Read the model definition and answer for the solid it produces. Units are mm, in the model's axes. A direction names the side the tool comes from. Round coordinates to 2 decimals unless told otherwise and drop trailing zeros. Write each loop counter-clockwise with the first axis right and the second up, starting at its lowest first coordinate (ties: lowest second). Pieces come first, ordered by that corner, then holes. Notation, with made-up numbers: (89.5, -12.75) -> (136.5, -12.75) arc R24 cw to (136.5, 25.25) -> close; hole circle Ø1 at (-20.75, 84.25). An arc over 180 degrees is marked (long way). Return JSON: item names as keys, results as strings.
from build123d import *

# Parameters (mm, degrees)
BOSS_EXTRUDE1_DEPTH = 15
SKETCH2_R           = 1.65
SKETCH2_W           = 4
SKETCH2_H           = 0.5
CUT_EXTRUDE1_DEPTH  = 9.2
SKETCH3_W           = 4.3
SKETCH3_H           = 5
CUT_EXTRUDE2_DEPTH  = 6


with BuildPart() as part:
    # Sketch1 → Boss-Extrude1 (new body)
    with BuildSketch(Plane.XY):
        Polygon((-3.803278689, 0), (4.196721311, 0), (4.196721311, 6.2), (2.887726083, 10), (-1.812273917, 10), (-3.803278689, 6.2), align=None)
    extrude(amount=BOSS_EXTRUDE1_DEPTH)

    # Sketch2 → Cut-Extrude1 (cut)
    with BuildSketch(Plane(origin=(0, 10, 0), x_dir=(1, 0, 0), z_dir=(0, 1, 0))):
        with Locations((0.537726083, -12.4)):
            Circle(SKETCH2_R)
        with Locations((0.537726083, -7.5)):
            Circle(SKETCH2_R)
        with Locations((0.537726083, -2.6)):
            Circle(SKETCH2_R)
        with Locations((0.537726083, -9.95)):
            Rectangle(SKETCH2_W, SKETCH2_H)
        with Locations((0.537726083, -5.05)):
            Rectangle(SKETCH2_W, SKETCH2_H)
    extrude(amount=-CUT_EXTRUDE1_DEPTH, mode=Mode.SUBTRACT)

    # Sketch3 → Cut-Extrude2 (cut)
    with BuildSketch(Plane(origin=(4.196721311, 0, 0), x_dir=(0, 0, -1), z_dir=(1, 0, 0))):
        with Locations((-12.4, 3.1)):
            Rectangle(SKETCH3_W, SKETCH3_H)
        with Locations((-7.5, 3.1)):
            Rectangle(SKETCH3_W, SKETCH3_H)
        with Locations((-2.6, 3.1)):
            Rectangle(SKETCH3_W, SKETCH3_H)
    extrude(amount=-CUT_EXTRUDE2_DEPTH, mode=Mode.SUBTRACT)


solid = part.part
Item 1: A flat-ended cylindrical pin translates along its axis: pin 1 (3 mm diameter, centred on x = 0.54, z = 2.6, fed in from +Y). Find the tip coordinate at first contact, or state that the pin passes through.
Worked answers:
{"pin 1": "stops at y = 0.6"}
Item 2: Section D-D (x = 3.5) is taken. Give the vertices of the cut face in (y, z), then the cut area to 3 significant figures.
Worked answers:
{"outline": "(0, 0) -> (8.22, 0) -> (8.22, 15) -> (0, 15) -> close; hole (0.6, 0.45) -> (5.6, 0.45) -> (5.6, 4.75) -> (0.6, 4.75) -> close; hole (0.6, 5.35) -> (5.6, 5.35) -> (5.6, 9.65) -> (0.6, 9.65) -> close; hole (0.6, 10.25) -> (5.6, 10.25) -> (5.6, 14.55) -> (0.6, 14.55) -> close", "area": "58.8 mm2"}
Item 3: For a pull along Z with two mould halves and no side action, classify faces 4 (the flat face through (-3.803, 3, 7)), 5 (the flat face through (-1.803, 3, 3)) as released by +Z, released by -Z, zero draft, split by the parting line, or undercut.
Worked answers:
{"face 4": "zero draft", "face 5": "undercut"}
Item 4: Section A-A (y = 1) is taken. Give the vertices of the cut face in (x, z), then the cut area to 3 significant figures.
Worked answers:
{"outline": "(-3.8, 0) -> (4.2, 0) -> (4.2, 0.45) -> (-1.8, 0.45) -> (-1.8, 4.75) -> (4.2, 4.75) -> (4.2, 5.35) -> (-1.8, 5.35) -> (-1.8, 9.65) -> (4.2, 9.65) -> (4.2, 10.25) -> (-1.8, 10.25) -> (-1.8, 14.55) -> (4.2, 14.55) -> (4.2, 15) -> (-3.8, 15) -> close; hole (-1.46, 4.8) -> (2.54, 4.8) -> (2.54, 5.3) -> (-1.46, 5.3) -> close; hole (-1.46, 9.7) -> (2.54, 9.7) -> (2.54, 10.2) -> (-1.46, 10.2) -> close", "area": "38.6 mm2"}
Item 5: Section B-B (z = 2.6) is taken. Give the vertices of the cut face in (x, y).
Worked answers:
{"outline": "(-3.8, 0) -> (4.2, 0) -> (4.2, 0.6) -> (-1.8, 0.6) -> (-1.8, 5.6) -> (-1.11, 5.6) -> (-1.11, 10) -> (-1.81, 10) -> (-3.8, 6.2) -> close; (2.19, 5.6) -> (4.2, 5.6) -> (4.2, 6.2) -> (2.89, 10) -> (2.19, 10) -> close"}
Item 6: Section C-C (y = 6) is taken. Give the vertices of the cut face in (x, z), then the cut area to 3 significant figures.
Worked answers:
{"outline": "(-3.8, 0) -> (4.2, 0) -> (4.2, 15) -> (-3.8, 15) -> close; hole (-1.46, 4.8) -> (2.54, 4.8) -> (2.54, 5.3) -> (-1.46, 5.3) -> close; hole (-1.46, 9.7) -> (2.54, 9.7) -> (2.54, 10.2) -> (-1.46, 10.2) -> close; hole circle Ø3.3 at (0.54, 2.6); hole circle Ø3.3 at (0.54, 7.5); hole circle Ø3.3 at (0.54, 12.4)", "area": "90.3 mm2"}
Item 7: Straight lines are drawn through the part: L1, parallel to Z at x = 2.75, y = 1; L2, parallel to Z at x = 0.5, y = 6.25; L3, parallel to Y at x = -1, z = 9.25. For each, find the intervals that lie inside material, in ascending order. Write a range as [from, to].
Worked answers:
{"L1": "z = [0, 0.45], [4.75, 5.35], [9.65, 10.25], [14.55, 15]", "L2": "z = [0, 0.95], [4.25, 4.8], [5.3, 5.85], [9.15, 9.7], [10.2, 10.75], [14.05, 15]", "L3": "y = [0, 0.6], [5.6, 10]"}
Item 8: A tool of negligible diameter and unlimited length cuts with its end or side. For faces 1 (the flat face through (0.6, 10, 5.7)), 2 (the flat face through (3, 5.6, 12)), 3 (the cylindrical face through (2.062, 7.831, 3.232)), from which of +Z, -Z, +X, -X, +Y, -Y can it reach the whole face along a straight path? Write none if from no direction.
Worked answers:
{"face 1": "+Z, -Z, +X, -X, +Y", "face 2": "+X", "face 3": "+Y"}
